Part model, mm, in its own coordinate system. A direction names the side the tool comes from. Coordinates: 2 decimals unless noted, no trailing zeros. Loops run counter-clockwise (first coordinate to the right, second up) from the corner with the lowest first, then second, coordinate; pieces in that order, holes last.
```python
from build123d import *

# Parameters (mm, degrees)
F0_W     = 223
F0_H     = 172
F0_W_2   = 189
F0_H_2   = 138
F0_W_3   = 173
F0_H_3   = 122
F1_DEPTH = 20
F2_SIZE  = 5
F3_DEPTH = 10


# Not quite as in the source:
# - a feature names something its author has since deleted; it is built from what else it names


with BuildPart() as f1:
    # F0 (on Front) → F1 (new body)
    with BuildSketch(Plane.XZ):
        Rectangle(F0_W, F0_H)
        Rectangle(F0_W_2, F0_H_2, mode=Mode.SUBTRACT)
        Rectangle(F0_W_2, F0_H_2)
        Rectangle(F0_W_3, F0_H_3, mode=Mode.SUBTRACT)
    extrude(amount=F1_DEPTH)

    # F2
    f2_edges = [f1.edges().sort_by_distance(p)[0] for p in [
        (-111.5, -20, 0),
        (0, -20, 86),
        (111.5, -20, 0),
        (0, -20, -86),
    ]]
    chamfer(f2_edges, length=F2_SIZE)

    # F0 (on Front) → F3 (cut)
    with BuildSketch(Plane.XZ):
        Rectangle(F0_W_2, F0_H_2)
        Rectangle(F0_W_3, F0_H_3, mode=Mode.SUBTRACT)
    extrude(amount=F3_DEPTH, mode=Mode.SUBTRACT)


solid = f1.part
```
Q1. Tool access for faces 4 (the flat face through (111.5, -7, -1)), 5 (the flat face through (86.5, -15, -1)), 6 (the flat face through (0, -10, -66)): list every direction of +Z, -Z, +X, -X, +Y, -Y with a clear straight run to the whole face (end or side of a thin tool).
Q2. Probe line 1 (X direction, y = -3.25, z = 57.5); line 2 (X direction, y = -10.75, z = -3); line 3 (Z direction, x = 72, y = -2.5). List the from-to ranges inside material, lowest first.
Q3. Saw through at A-A (x = -62). List the corners of the cut face in (y, z), plus the area to 3 significant figures.
Q4. Saw through at B-B (z = -36). List the corners of the cut face in (x, y), plus the area to 3 significant figures.
Q5. Drop a flat-ended pin along its axis: P1, Ø3, axis at x = -3.5, y = -16, coming from the -Z side. Give the stop position or say it passes through.
Q6. Saw through at C-C (y = -6.5). List the corners of the cut face in (x, z).
Q7. Mould opens along Z. For faces 1 (the flat face through (-2, -18, 83)), 2 (the flat face through (94.5, -5, -1)), 3 (the flat face through (-1, -20, -71)) say: released by +Z, released by -Z, zero draft, split by the parting line, or undercut.
Checked values:
1. face 4: +Z, -Z, +X, +Y, -Y
1. face 5: +Y, -Y
1. face 6: +Y
2. line 1: x = -111.5 to -94.5, 94.5 to 111.5
2. line 2: x = -111.5 to -86.5, 86.5 to 111.5
2. line 3: z = -86 to -69, 69 to 86
3. outline: (-20, -81) - (-15, -86) - (0, -86) - (0, -69) - (-10, -69) - (-10, -61) - (-20, -61) - close; (-20, 61) - (-10, 61) - (-10, 69) - (0, 69) - (0, 86) - (-15, 86) - (-20, 81) - close
3. area: 815 mm2
4. outline: (-111.5, -15) - (-106.5, -20) - (-86.5, -20) - (-86.5, -10) - (-94.5, -10) - (-94.5, 0) - (-111.5, 0) - close; (86.5, -20) - (106.5, -20) - (111.5, -15) - (111.5, 0) - (94.5, 0) - (94.5, -10) - (86.5, -10) - close
4. area: 815 mm2
5. P1: stops at z = -86
6. outline: (-111.5, -86) - (111.5, -86) - (111.5, 86) - (-111.5, 86) - close; hole (-94.5, -69) - (94.5, -69) - (94.5, 69) - (-94.5, 69) - close
7. face 1: released by +Z
7. face 2: undercut
7. face 3: zero draft
